For this review, take the finished solid that the model builds, in its own axes (mm). A direction names the side the tool comes from. Coordinates: 2 decimals unless noted, no trailing zeros. Order: outer loops, then holes, each group sorted by start corner. A loop starts at its lowest first (then second) coordinate and runs counter-clockwise, first axis right, second up. Notation, with made-up numbers: M -8,-24.5 L 20,-24.5 A26 cw 20,5.5 Z; hole C 76,11.5 d7. An arc over 180 degrees is marked long. Use one line per item in the form item = value. Start each with the question number.
Autodesk Inventor part; units mm, degrees
ref_plane "YZ Plane" through (0, 0, 0) normal (1, 0, 0) x (0, 1, 0)
ref_plane "XZ Plane" through (0, 0, 0) normal (0, 1, 0) x (-1, 0, 0)
ref_plane "XY Plane" through (0, 0, 0) normal (0, 0, 1) x (1, 0, 0)
sketch "Sketch1" plane through (0, 0, 0) normal (0, 1, 0) x (-1, 0, 0)
  circle A0 centre (0, 0) radius 12.7
  circle A1 centre (0, 0) radius 25.4
  line L0 (-12.7, -21.997) -> (-95.25, -21.997)
  line L1 (-95.25, 21.997) -> (-12.7, 21.997)
  arc A2 (-63.5, -9.525) -> (-63.5, 9.525) centre (-63.5, 0) ccw
  line L2 (-63.5, 9.525) -> (-95.25, 9.525)
  line L3 (-78.5703, 0) -> (-63.5, 0) construction
  line L4 (-63.5, -9.525) -> (-95.25, -9.525)
  line L5 (-95.25, -21.997) -> (-95.25, -9.525)
  line L6 (-95.25, 9.525) -> (-95.25, 21.997)
  line L7 (-44.45, 21.997) -> (-44.45, 12.472)
  line L8 (-44.45, 12.472) -> (-22.1271, 12.472)
  line L9 (-52.07, 21.997) -> (-52.07, -21.997)
  dimension "d0" = 25.4
  dimension "d3" = 19.05
  dimension "d4" = 31.75
  dimension "d5" = 12.7
  dimension "d6" = 44.45
  dimension "d7" = 9.525
  dimension "d8" = 7.62
  dimension "d9" = 82.55
  dimension "d10" = 12.7
extrude "Extrusion3" add sketch "Sketch1" along normal blind 50.8 contours A1
extrude "Extrusion4" add sketch "Sketch1" along normal blind 6.35 contours A1 L8 L7 L1 | L0 L9 L1 L7 L8 A1 | L0 L5 L4 A2 L2 L6 L1 L9
extrude "Extrusion5" add sketch "Sketch1" along normal blind 6.35 from surface at 6.35 contours A1 L8 L7 L1 | L0 L9 L1 L7 L8 A1
extrude "Extrusion6" add sketch "Sketch1" along normal blind 25.4 from surface at 12.7 contours A1 L8 L7 L1
properties part number "Distance from Face Complete"
1. Consider section B-B, the plane x = 80.5. Write out the cut boundary in (y, z) (3 decimals).
2. Consider section C-C, the plane y = 4. Write out the cut boundary in (x, z) (3 decimals), plus the area to 3 significant figures.
3. Tool access review of faces 1 (the flat face through (44.45, 25, 17)), 2 (the flat face through (79, 3, -9.525)), 3 (the flat face through (32, 38.1, 17)), 4 (the flat face through (36, 15, 21.997)): name each direction out of +Z, -Z, +X, -X, +Y, -Y from which nothing blocks a thin tool from reaching the whole face with its end or side.
4. For pin 1 Ø7.5 at (y, z) = (31.5, 17.5) entering from +X; pin 2 Ø23 at (x, z) = (0, 0) entering from -Y; pin 3 Ø3 at (x, y) = (82, 2.5) entering from +Z; pin 4 Ø14 at (x, y) = (62.5, 4.5) entering from -Z, all flat-tipped, find the tip position at first contact; note any pin that passes through.
5. To check wall thickness, follow line 1 (Z direction, x = 0, y = 14.5); line 2 (Y direction, x = 35.5, z = -2); line 3 (Z direction, x = 4.5, y = 2.5). State the ranges of each line that lie inside material, in increasing order.
6. Consider section A-A, the plane z = 0. Write out the cut boundary in (x, y) (3 decimals), plus the area to 3 significant figures.
7. The part is to be moulded in two halves that separate along X. For faces 5 (the cylindrical face through (-24.227, 25.044, -7.629)), 6 (the cylindrical face through (2.75, 25.04, 12.4)), 7 (the flat face through (95.25, 3, 16)), 8 (the flat face through (-5, 50.8, 12)), say which applies: pulls with the +X half, pulls with the -X half, needs draft (parallel to the pull), parting line crosses it, or undercut.
8. Consider section D-D, the plane x = 5. Write out the cut boundary in (y, z), plus the area to 3 significant figures.
Answers follow:
q1.outline = M 0,-21.997 L 6.35,-21.997 L 6.35,-9.525 L 0,-9.525 Z; M 0,9.525 L 6.35,9.525 L 6.35,21.997 L 0,21.997 Z
q2.outline = M 12.7,-21.997 L 95.25,-21.997 L 95.25,-9.525 L 63.5,-9.525 A9.525 cw 63.5,9.525 L 95.25,9.525 L 95.25,21.997 L 12.7,21.997 A25.4 ccw long Z; hole C 0,0 d25.4
q2.area = 4,010 mm²
q3.face_1 = +Z, -Z, +X, +Y
q3.face_2 = +X, +Y, -Y
q3.face_3 = +Z, +X, +Y
q3.face_4 = +Z, +X, +Y, -Y
q4.pin_1 = 44.45
q4.pin_2 = through
q4.pin_3 = 22
q4.pin_4 = -22
q5.line_1 = -25.4 to -12.7, 12.7 to 25.4
q5.line_2 = 0 to 12.7
q5.line_3 = -25 to -11.88, 11.88 to 25
q6.outline = M -25.4,0 L -12.7,0 L -12.7,50.8 L -25.4,50.8 Z; M 12.7,0 L 53.975,0 L 53.975,6.35 L 52.07,6.35 L 52.07,12.7 L 25.4,12.7 L 25.4,50.8 L 12.7,50.8 Z
q6.area = 1,640 mm²
q7.face_5 = parting line crosses it
q7.face_6 = undercut
q7.face_7 = pulls with the +X half
q7.face_8 = needs draft
q8.outline = M 0,-24.9 L 50.8,-24.9 L 50.8,-11.67 L 0,-11.67 Z; M 0,11.67 L 50.8,11.67 L 50.8,24.9 L 0,24.9 Z
q8.area = 1,340 mm²
